```python
from build123d import *

# Parameters (mm, degrees)
F0_R     = 9.5
F1_DEPTH = 37
F2_R     = 7
F3_DEPTH = 36
F2_R_2   = 8.55
F4_DEPTH = 12


with BuildPart() as f1:
    # F0 (on Top) → F1 (new body)
    with BuildSketch(Plane.XY):
        Circle(F0_R)
    extrude(amount=F1_DEPTH)

    # F2 (on face) → F3 (cut)
    with BuildSketch(Plane.XY.offset(37)):
        Circle(F2_R)
    extrude(amount=-F3_DEPTH, mode=Mode.SUBTRACT)

    # F2 (on face) → F4 (cut)
    with BuildSketch(Plane.XY.offset(37)):
        Circle(F2_R_2)
        Circle(F2_R, mode=Mode.SUBTRACT)
    extrude(amount=-F4_DEPTH, mode=Mode.SUBTRACT)


solid = f1.part
```
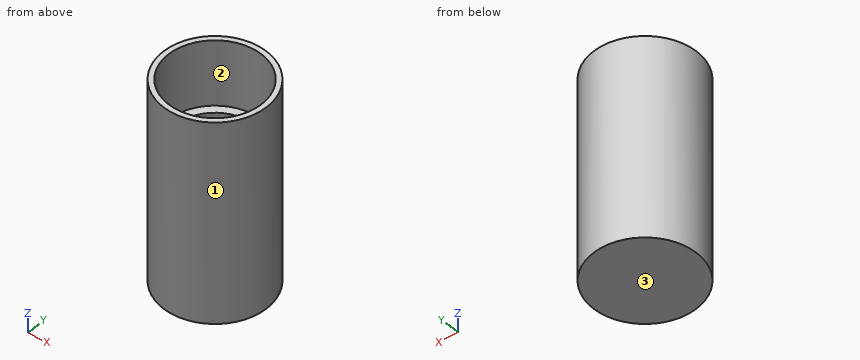
Can you work these out from the model? Positions are in its coordinate system, mm. Face numbers are marked on the shaded views. Coordinates: 2 decimals unless noted, no trailing zeros. Order: outer loops, then holes, each group sorted by start corner. A loop starts at its lowest first (then second) coordinate and runs counter-clockwise, first axis right, second up.
1. Thinking about a two-plate mould opening in X: for the marked faces 1, 2 and 3, which applies, +X half, -X half, draft (parallel to the pull), parting line (faces both ways), or undercut?
2. I'm going to push flat-ended pins straight in: pin 1 (5 mm diameter, centred on x = 3.5, y = 1.5, fed in from +Z); pin 2 (2 mm diameter, centred on y = 5, z = 21.5, fed in from -X); pin 3 (1 mm diameter, centred on y = 3, z = 22, fed in from +X). Where does each tip first touch, or does it pass through?
3. If we section it at A-A (x = 0): Please give me the cut outline in (y, z), then the cut area to 3 significant figures.
4. If we section it at B-B (z = 3.5): Please give me the cut outline in (x, y), then the cut area to 3 significant figures.
5. I need wall thicknesses on line 1 (Y direction, x = 0, z = 15); line 2 (Y direction, x = 0, z = 34.5); line 3 (Z direction, x = -2.75, y = -1). Which ranges of each line are inside material? Lowest first, please.
6. If we section it at D-D (z = 26): Please give me the cut outline in (x, y), then the cut area to 3 significant figures.
Entries:
1. face 1: parting line
1. face 2: undercut
1. face 3: draft
2. pin 1: stops at z = 1
2. pin 2: stops at x = -8.62
2. pin 3: stops at x = 9.17
3. outline: (-9.5, 0) - (9.5, 0) - (9.5, 37) - (8.55, 37) - (8.55, 25) - (7, 25) - (7, 1) - (-7, 1) - (-7, 25) - (-8.55, 25) - (-8.55, 37) - (-9.5, 37) - close
3. area: 162 mm2
4. outline: circle Ø19 at (0, 0); hole circle Ø14 at (0, 0)
4. area: 130 mm2
5. line 1: y = -9.5 to -7, 7 to 9.5
5. line 2: y = -9.5 to -8.55, 8.55 to 9.5
5. line 3: z = 0 to 1
6. outline: circle Ø19 at (0, 0); hole circle Ø17.1 at (0, 0)
6. area: 53.9 mm2
